Part model, mm, in its own coordinate system. Face numbers are marked on the shaded views. A direction names the side the tool comes from. Round coordinates to 2 decimals unless told otherwise and drop trailing zeros. Write each loop counter-clockwise with the first axis right and the second up, starting at its lowest first coordinate (ties: lowest second). Pieces come first, ordered by that corner, then holes. Notation, with made-up numbers: (-11, 52.5) -> (35, 52.5) arc R21 cw to (35, 56.5) -> close; hole circle Ø2 at (25, 37.25). An arc over 180 degrees is marked (long way). Return JSON: item names as keys, results as strings. Group by question number.
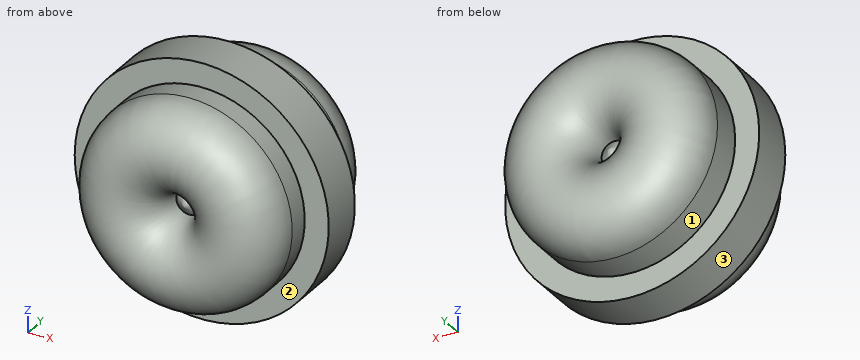
```python
from build123d import *

# Parameters (mm, degrees)
F0_W = 12.0748467743
F0_H = 22.6198285818


with BuildPart() as f1:
    # F0 (on Top) → F1 (revolve)
    with BuildSketch(Plane.XY):
        with BuildLine():
            ThreePointArc((-51.7385564744, -24.759542197), (-29.1173150763, -47.3807835951), (-6.4960736781, -24.759542197))
            Line((-6.4960736781, -24.759542197), (-51.7385564744, -24.759542197))
        make_face()
        with BuildLine():
            Line((-51.7385564744, 23.9953603595), (-6.4960736781, 23.9953603595))
            ThreePointArc((-6.4960736781, 23.9953603595), (-29.1173150763, 46.6166017577), (-51.7385564744, 23.9953603595))
        make_face()
        Polygon((-6.4960736781, 23.9953603595), (-6.4960736781, -24.759542197), (0, -29.3446425349), (0, 28.4276213497), align=None)
        with Locations((-57.7759798616, -2.5982232764)):
            Rectangle(F0_W, F0_H)
        Polygon((-51.7385564744, -24.759542197), (-6.4960736781, -24.759542197), (-6.4960736781, 23.9953603595), (-51.7385564744, 23.9953603595), (-51.7385564744, 8.7116910145), (-51.7385564744, -13.9081375673), align=None)
    revolve(axis=Axis((0, -0.4585105926, 0), (0, 1, 0)))


solid = f1.part
```
Item 1: Cut at A-A (y = 12). Write the cut outline in (x, z).
Item 2: Flat gauge pins, fed straight in: P1, Ø3, axis at y = -0.5, z = 39.5, coming from the -X side; P2, Ø1.5, axis at x = 45, z = 16.5, coming from the -Y side; P3, Ø12, axis at x = -35.5, z = -17.5, coming from the +Y side. Where does each tip first touch, or does it go through?
Item 3: Which spindle directions (+Z, -Z, +X, -X, +Y, -Y) get a long thin tool onto all of the face, cutting with end or side? Do the marked faces 1, 2 and 3. Say none if no direction does.
Item 4: Wall check: L1, parallel to X at y = -40, z = -3; L2, parallel to Y at x = -13, z = 27; L3, parallel to Y at x = -12, z = 54. Give the ranges that are in metal, low to high.
Item 5: Cut at B-B (y = 36). Write the cut outline in (x, z).
Checks:
{
 "1": {"outline": "circle Ø103.48 at (0, 0)"},
 "2": {"P1": "stops at x = -51.27", "P2": "stops at y = -38.38", "P3": "stops at y = 46.17"},
 "3": {"face 1": "+Y", "face 2": "-Y", "face 3": "+Y, -Y"},
 "4": {"L1": "x = -45.74 to -12.03, 12.03 to 45.74", "L2": "y = -47.36 to 46.6", "L3": "y = -13.91 to 8.71"},
 "5": {"outline": "circle Ø96.58 at (0, 0); hole circle Ø19.89 at (0, 0)"}
}
